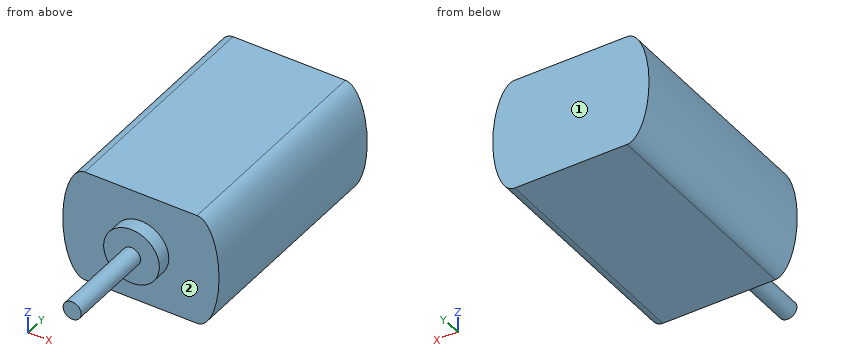
from build123d import *

# Parameters (mm, degrees)
SKETCH2_RX          = 6.2
SKETCH2_RY          = 2.428962841
SKETCH2_RY_2        = 2.417240448
SKETCH2_W           = 12.4
SKETCH2_H           = 12.4
BOSS_EXTRUDE1_DEPTH = 25.1
SKETCH3_R           = 3.075
BOSS_EXTRUDE2_DEPTH = 1.6
SKETCH4_R           = 1
BOSS_EXTRUDE3_DEPTH = 10.05


with BuildPart() as part:
    # Sketch2 → Boss-Extrude1 (new body)
    with BuildSketch(Plane(origin=(0, 0, 0), x_dir=(1, 0, 0), z_dir=(0, 1, 0))):
        with Locations(Location((-6.2, 0), (0, 0, -90))):
            Ellipse(SKETCH2_RX, SKETCH2_RY)
        with Locations(Location((6.2, 0), (0, 0, -90))):
            Ellipse(SKETCH2_RX, SKETCH2_RY_2)
        Rectangle(SKETCH2_W, SKETCH2_H)
    extrude(amount=BOSS_EXTRUDE1_DEPTH)

    # Sketch3 → Boss-Extrude2 (add)
    with BuildSketch(Plane.XZ):
        with Locations(Location((0, 0, 0), (0, 0, 270))):
            Circle(SKETCH3_R)
    extrude(amount=BOSS_EXTRUDE2_DEPTH)

    # Sketch4 → Boss-Extrude3 (add)
    with BuildSketch(Plane.XZ.offset(1.6)):
        with Locations(Location((0, 0, 0), (0, 0, 270))):
            Circle(SKETCH4_R)
    extrude(amount=BOSS_EXTRUDE3_DEPTH)


solid = part.part
Work out the finished part from the listing and answer in its coordinate system (mm). Face numbers are marked on the shaded views. A direction names the side the tool comes from. Give positions to 0.01 mm unless a question says otherwise; leave off trailing zeros. Write each loop counter-clockwise with the first axis right and the second up, starting at its lowest first coordinate (ties: lowest second). Pieces come first, ordered by that corner, then holes. Notation, with made-up numbers: (50, 31) - (58, 31) arc R34 cw to (58, 68) - close; hole circle Ø7 at (34.25, -35). An arc over 180 degrees is marked (long way). One line per item, written item: value. Start each with the question number.
1. Find section A-A (x = 0). Write down the section's boundary in (y, z) (3 decimals).
2. For the marked faces 1 and 2, determine the directions among +Z, -Z, +X, -X, +Y, -Y from which every point of the face is accessible in a straight line to the end or side of a thin tool.
3. Find section B-B (y = -8). Write down the section's boundary in (x, z).
4. Find section C-C (x = -4). Write down the section's boundary in (y, z), then the cut area to 3 significant figures.
5. Find section D-D (x = 2.25). Write down the section's boundary in (y, z), then the cut area to 3 significant figures.
6. Consider probe 1 along Y at (x, z) = (-3, -0.25); probe 2 along Y at (x, z) = (3.75, 3); probe 3 along X at (y, z) = (16, 5.25). Determine where each line is inside the solid, lowest interval first.
7. Given pin 1 (6 mm diameter, centred on x = -0.5, z = 1.5, fed in from -Y); pin 2 (1 mm diameter, centred on x = 0, z = 4.5, fed in from -Y); pin 3 (1 mm diameter, centred on y = 2.5, z = -4, fed in from -X); pin 4 (1 mm diameter, centred on y = 19.5, z = 3, fed in from -X), each flat-ended and moving along its own axis, determine where each tip first touches the part or whether it passes through.
Geometry results:
1. outline: (-11.65, -1) - (-1.6, -1) - (-1.6, -3.075) - (0, -3.075) - (0, -6.2) - (25.1, -6.2) - (25.1, 6.2) - (0, 6.2) - (0, 3.075) - (-1.6, 3.075) - (-1.6, 1) - (-11.65, 1) - close
2. face 1: +Z, -Z, +X, -X, +Y
2. face 2: -Y
3. outline: circle Ø2 at (0, 0)
4. outline: (0, -6.2) - (25.1, -6.2) - (25.1, 6.2) - (0, 6.2) - close
4. area: 311 mm2
5. outline: (-1.6, -2.1) - (0, -2.1) - (0, -6.2) - (25.1, -6.2) - (25.1, 6.2) - (0, 6.2) - (0, 2.1) - (-1.6, 2.1) - close
5. area: 318 mm2
6. probe 1: -1.6 to 25.1
6. probe 2: 0 to 25.1
6. probe 3: -7.49 to 7.49
7. pin 1: y = -11.65
7. pin 2: y = 0
7. pin 3: x = -8.2
7. pin 4: x = -8.42
